```python
from build123d import *

# Parameters (mm, degrees)
SKETCH_1_R           = 1.75
EXTRUDE_3_DEPTH      = 3
EXTRUDE_4_DEPTH      = 15
SKETCH_3_R           = 1
CUT_EXTRUDE_5_DEPTH  = 7.5
SKETCH_8_R           = 0.85
CUT_EXTRUDE_8_DEPTH  = 9
SKETCH_10_R          = 0.85
CUT_EXTRUDE_9_DEPTH  = 9
SKETCH_11_R          = 0.85
CUT_EXTRUDE_10_DEPTH = 9
SKETCH_12_R          = 0.85
CUT_EXTRUDE_11_DEPTH = 9
SKETCH_13_R          = 2
SKETCH_13_R_2        = 0.85
EXTRUDE_5_DEPTH      = 10
SKETCH_14_R          = 2
SKETCH_14_R_2        = 0.85
EXTRUDE_6_DEPTH      = 10
SKETCH_15_R          = 2
SKETCH_15_R_2        = 0.85
EXTRUDE_7_DEPTH      = 10
SKETCH_16_R          = 2
SKETCH_16_R_2        = 0.85
EXTRUDE_8_DEPTH      = 10
SKETCH_17_R          = 4
SKETCH_17_R_2        = 2
EXTRUDE_9_DEPTH      = 8
SKETCH_18_R          = 1.75
EXTRUDE_10_DEPTH     = 3
SKETCH_19_R          = 2
EXTRUDE_11_DEPTH     = 3


with BuildPart() as part:
    # 草图1 → 凸台-拉伸3 (new body)
    with BuildSketch(Plane.XY):
        with BuildLine():
            Line((-18, -25), (18, -25))
            ThreePointArc((18, -25), (22.949747468, -22.949747468), (25, -18))
            Line((25, -18), (25, 18))
            ThreePointArc((25, 18), (22.949747468, 22.949747468), (18, 25))
            Line((18, 25), (-18, 25))
            ThreePointArc((-18, 25), (-22.949747468, 22.949747468), (-25, 18))
            Line((-25, 18), (-25, -18))
            ThreePointArc((-25, -18), (-22.949747468, -22.949747468), (-18, -25))
        make_face()
        with Locations((20, 20)):
            Circle(SKETCH_1_R, mode=Mode.SUBTRACT)
        with Locations((-20, 20)):
            Circle(SKETCH_1_R, mode=Mode.SUBTRACT)
        with Locations((-20, -20)):
            Circle(SKETCH_1_R, mode=Mode.SUBTRACT)
        with Locations((20, -20)):
            Circle(SKETCH_1_R, mode=Mode.SUBTRACT)
    extrude(amount=EXTRUDE_3_DEPTH)

    # 草图2 → 凸台-拉伸4 (add)
    with BuildSketch(Plane(origin=(0, 0, 0), x_dir=(-1, 0, 0), z_dir=(0, 0, -1))):
        Polygon((9.814954576, -17), (19.629909152, 0), (9.814954576, 17), (-9.814954576, 17), (-19.629909152, 0), (-9.814954576, -17), align=None)
    extrude(amount=EXTRUDE_4_DEPTH)

    # 草图3 → 切除-拉伸5 (cut)
    with BuildSketch(Plane(origin=(0, 0, -15), x_dir=(-1, 0, 0), z_dir=(0, 0, -1))):
        with Locations((-4.815101245, 8.34)):
            Circle(SKETCH_3_R)
        with Locations((4.815101245, 8.34)):
            Circle(SKETCH_3_R)
        with Locations((4.815101245, -8.34)):
            Circle(SKETCH_3_R)
        with Locations((-4.815101245, -8.34)):
            Circle(SKETCH_3_R)
    extrude(amount=-CUT_EXTRUDE_5_DEPTH, mode=Mode.SUBTRACT)

    # 草图8 → 切除-拉伸8 (cut)
    with BuildSketch(Plane(origin=(14.722431864, 8.5, 0), x_dir=(0, 0, -1), z_dir=(0.866025404, 0.5, 0))):
        with Locations((10, 4.814954576)):
            Circle(SKETCH_8_R)
    extrude(amount=-CUT_EXTRUDE_8_DEPTH, mode=Mode.SUBTRACT)

    # 草图10 → 切除-拉伸9 (cut)
    with BuildSketch(Plane(origin=(-14.722431864, 8.5, 0), x_dir=(0, 0, 1), z_dir=(-0.866025404, 0.5, 0))):
        with Locations((-10, 4.814954576)):
            Circle(SKETCH_10_R)
    extrude(amount=-CUT_EXTRUDE_9_DEPTH, mode=Mode.SUBTRACT)

    # 草图11 → 切除-拉伸10 (cut)
    with BuildSketch(Plane(origin=(-14.722431864, -8.5, 0), x_dir=(0, 0, 1), z_dir=(-0.866025404, -0.5, 0))):
        with Locations((-10, -4.814954576)):
            Circle(SKETCH_11_R)
    extrude(amount=-CUT_EXTRUDE_10_DEPTH, mode=Mode.SUBTRACT)

    # 草图12 → 切除-拉伸11 (cut)
    with BuildSketch(Plane(origin=(14.722431864, -8.5, 0), x_dir=(0, 0, -1), z_dir=(0.866025404, -0.5, 0))):
        with Locations((10, -4.814954576)):
            Circle(SKETCH_12_R)
    extrude(amount=-CUT_EXTRUDE_11_DEPTH, mode=Mode.SUBTRACT)

    # 草图13 → 凸台-拉伸5 (add)
    with BuildSketch(Plane(origin=(14.722431864, 8.5, 0), x_dir=(0, 0, -1), z_dir=(0.866025404, 0.5, 0))):
        with Locations((10, 4.814954576)):
            Circle(SKETCH_13_R)
        with Locations((10, 4.814954576)):
            Circle(SKETCH_13_R_2, mode=Mode.SUBTRACT)
    extrude(amount=EXTRUDE_5_DEPTH)

    # 草图14 → 凸台-拉伸6 (add)
    with BuildSketch(Plane(origin=(-14.722431864, 8.5, 0), x_dir=(0, 0, 1), z_dir=(-0.866025404, 0.5, 0))):
        with Locations((-10, 4.814954576)):
            Circle(SKETCH_14_R)
        with Locations((-10, 4.814954576)):
            Circle(SKETCH_14_R_2, mode=Mode.SUBTRACT)
    extrude(amount=EXTRUDE_6_DEPTH)

    # 草图15 → 凸台-拉伸7 (add)
    with BuildSketch(Plane(origin=(-14.722431864, -8.5, 0), x_dir=(0, 0, 1), z_dir=(-0.866025404, -0.5, 0))):
        with Locations((-10, -4.814954576)):
            Circle(SKETCH_15_R)
        with Locations((-10, -4.814954576)):
            Circle(SKETCH_15_R_2, mode=Mode.SUBTRACT)
    extrude(amount=EXTRUDE_7_DEPTH)

    # 草图16 → 凸台-拉伸8 (add)
    with BuildSketch(Plane(origin=(14.722431864, -8.5, 0), x_dir=(0, 0, -1), z_dir=(0.866025404, -0.5, 0))):
        with Locations((10, -4.814954576)):
            Circle(SKETCH_16_R)
        with Locations((10, -4.814954576)):
            Circle(SKETCH_16_R_2, mode=Mode.SUBTRACT)
    extrude(amount=EXTRUDE_8_DEPTH)

    # 草图17 → 凸台-拉伸9 (add)
    with BuildSketch(Plane(origin=(0, 0, -15), x_dir=(-1, 0, 0), z_dir=(0, 0, -1))):
        with Locations((4.815101245, 8.34)):
            Circle(SKETCH_17_R)
        with Locations((4.815101245, 8.34)):
            Circle(SKETCH_17_R_2, mode=Mode.SUBTRACT)
        with Locations((-4.815101245, 8.34)):
            Circle(SKETCH_17_R)
        with Locations((-4.815101245, 8.34)):
            Circle(SKETCH_17_R_2, mode=Mode.SUBTRACT)
        with Locations((-4.815101245, -8.34)):
            Circle(SKETCH_17_R)
        with Locations((-4.815101245, -8.34)):
            Circle(SKETCH_17_R_2, mode=Mode.SUBTRACT)
        with Locations((4.815101245, -8.34)):
            Circle(SKETCH_17_R)
        with Locations((4.815101245, -8.34)):
            Circle(SKETCH_17_R_2, mode=Mode.SUBTRACT)
    extrude(amount=EXTRUDE_9_DEPTH)

    # 草图18 → 凸台-拉伸10 (add)
    with BuildSketch(Plane(origin=(0, 0, 0), x_dir=(-1, 0, 0), z_dir=(0, 0, -1))):
        with Locations((20, 20)):
            Circle(SKETCH_18_R)
        with Locations((-20, 20)):
            Circle(SKETCH_18_R)
        with Locations((-20, -20)):
            Circle(SKETCH_18_R)
        with Locations((20, -20)):
            Circle(SKETCH_18_R)
    extrude(amount=-EXTRUDE_10_DEPTH)

    # 草图19 → 凸台-拉伸11 (add)
    with BuildSketch(Plane(origin=(0, 0, 0), x_dir=(-1, 0, 0), z_dir=(0, 0, -1))):
        with BuildLine():
            Line((-25, 35), (25, 35))
            ThreePointArc((25, 35), (32.071067812, 32.071067812), (35, 25))
            Line((35, 25), (35, -25))
            ThreePointArc((35, -25), (32.071067812, -32.071067812), (25, -35))
            Line((25, -35), (-25, -35))
            ThreePointArc((-25, -35), (-32.071067812, -32.071067812), (-35, -25))
            Line((-35, -25), (-35, 25))
            ThreePointArc((-35, 25), (-32.071067812, 32.071067812), (-25, 35))
        make_face()
        with Locations((-30, 5)):
            Circle(SKETCH_19_R, mode=Mode.SUBTRACT)
        with Locations((-30, -5)):
            Circle(SKETCH_19_R, mode=Mode.SUBTRACT)
        with Locations((-5, -30)):
            Circle(SKETCH_19_R, mode=Mode.SUBTRACT)
        with Locations((5, -30)):
            Circle(SKETCH_19_R, mode=Mode.SUBTRACT)
        with Locations((-5, 30)):
            Circle(SKETCH_19_R, mode=Mode.SUBTRACT)
        with Locations((5, 30)):
            Circle(SKETCH_19_R, mode=Mode.SUBTRACT)
        with Locations((30, 5)):
            Circle(SKETCH_19_R, mode=Mode.SUBTRACT)
        with Locations((30, -5)):
            Circle(SKETCH_19_R, mode=Mode.SUBTRACT)
    extrude(amount=-EXTRUDE_11_DEPTH)


solid = part.part
```
Check sheet for the modelled part. Datum: model origin and axes. Units: mm. A direction names the side the tool comes from. Coordinates: 2 decimals unless noted, no trailing zeros. Order: outer loops, then holes, each group sorted by start corner. A loop starts at its lowest first (then second) coordinate and runs counter-clockwise, first axis right, second up. Notation, with made-up numbers: M 52.25,45.5 L 104.25,45.5 A29 cw 104.25,78.5 Z; hole C -28.75,72.25 d5. An arc over 180 degrees is marked long. One line per question, with ' | ' between items. Start each with the question number.
Item 1: Mould release check, pull along Y, two halves, no side actions. Record for faces 3 (the cylindrical face through (-31.99, 32.15, 1.48)), 4 (the flat face through (-3, -7, -23)), 5 (the flat face through (6, 8, -15)): pulls with the +Y half, pulls with the -Y half, needs draft (parallel to the pull), parting line crosses it, or undercut.
Item 2: Access from +Z, -Z, +X, -X, +Y, -Y to the whole of each face (thin tool, end or side, straight path). Record for faces 1 (the flat face through (35, 0, 1)), 2 (the flat face through (-5, -7, -15)).
Item 3: Sectioned sample at A-A on z = -19.25. Record the cut outline in (x, y), and give its area (3 significant figures).
Item 4: Sectioned sample at C-C on x = 30. Record the cut outline in (y, z).
Item 5: Sectioned sample at B-B on y = 29. Record the cut outline in (x, z).
Item 6: Gauge pin test, flat ends, axial feed: P1, Ø1, axis at x = 9, y = 0.5, coming from the -Z side; P2, Ø1, axis at y = -11.5, z = -14, coming from the -X side; P3, Ø1.8, axis at x = 4.82, y = -8.34, coming from the -Z side; P4, Ø4.5, axis at x = 30, y = 5, coming from the +Z side. Record the tip position at first contact, or that the pin passes through.
Item 7: Sectioned sample at D-D on x = 14. Count the separate pieces of the cut face and the enclosed holes in it, and give its area (3 significant figures).
Item 8: Material ranges on line 1 (X direction, y = -9.5, z = -21.5); line 2 (Y direction, x = -30, z = 0.65); line 3 (Z direction, x = 19, y = -27), recorded low to high.
Answer below:
1) face 3: pulls with the +Y half | face 4: needs draft | face 5: undercut
2) face 1: +Z, -Z, +X, +Y, -Y | face 2: -Z
3) outline: C -4.82,-8.34 d8; C -4.82,8.34 d8; C 4.82,-8.34 d8; C 4.82,8.34 d8; hole C -4.82,-8.34 d4; hole C -4.82,8.34 d4; hole C 4.82,-8.34 d4; hole C 4.82,8.34 d4 | area: 151 mm^2
4) outline: M -33.66,0 L -7,0 L -7,3 L -33.66,3 Z; M -3,0 L 3,0 L 3,3 L -3,3 Z; M 7,0 L 33.66,0 L 33.66,3 L 7,3 Z
5) outline: M -34.17,0 L -6.73,0 L -6.73,3 L -34.17,3 Z; M -3.27,0 L 3.27,0 L 3.27,3 L -3.27,3 Z; M 6.73,0 L 34.17,0 L 34.17,3 L 6.73,3 Z
6) P1: stops at z = -15 | P2: stops at x = -13.28 | P3: stops at z = -7.5 | P4: stops at z = 3
7) separate pieces: 3 | enclosed holes: 2 | area: 526 mm^2
8) line 1: x = -8.64 to -6.44, -3.19 to -0.99, 0.99 to 3.19, 6.44 to 8.64 | line 2: y = -33.66 to -7, -3 to 3, 7 to 33.66 | line 3: z = 0 to 3
